Design review of the part built by this model. Coordinates are the model's own, in mm. Face numbers are marked on the shaded views. A direction names the side the tool comes from. Coordinates: 2 decimals unless noted, no trailing zeros. Write each loop counter-clockwise with the first axis right and the second up, starting at its lowest first coordinate (ties: lowest second). Pieces come first, ordered by that corner, then holes. Notation, with made-up numbers: (-23.5, 15.25) - (21.5, 15.25) arc R31 ccw to (21.5, 51.25) - close; hole circle Ø2 at (-33, -25). An arc over 180 degrees is marked (long way). Use a Markdown table: item, result.
from build123d import *

# Parameters (mm, degrees)
SKETCH1_W           = 30
SKETCH1_H           = 28
BOSS_EXTRUDE1_DEPTH = 20
SKETCH2_W           = 5
SKETCH2_H           = 28
BOSS_EXTRUDE2_DEPTH = 12
SKETCH3_W           = 3
SKETCH3_H           = 2
CUT_EXTRUDE1_DEPTH  = 53.038447325
SKETCH4_W           = 20
SKETCH4_H           = 20
CUT_EXTRUDE2_DEPTH  = 14
SKETCH5_W           = 7
SKETCH5_H           = 2
BOSS_EXTRUDE3_DEPTH = 28
FILLET1_R           = 2
BOSS_EXTRUDE5_DEPTH = 10
SKETCH8_W           = 26
SKETCH8_H           = 2
BOSS_EXTRUDE6_DEPTH = 8.8
BOSS_EXTRUDE7_DEPTH = 4


with BuildPart() as part:
    # Sketch1 → Boss-Extrude1 (new body)
    with BuildSketch(Plane(origin=(0, 0, 0), x_dir=(1, 0, 0), z_dir=(0, 1, 0))):
        with Locations((-15, 14)):
            Rectangle(SKETCH1_W, SKETCH1_H)
    extrude(amount=BOSS_EXTRUDE1_DEPTH)

    # Sketch2 → Boss-Extrude2 (add)
    with BuildSketch(Plane(origin=(0, 20, 0), x_dir=(1, 0, 0), z_dir=(0, 1, 0))):
        with Locations((-27.5, 14)):
            Rectangle(SKETCH2_W, SKETCH2_H)
        with Locations((-2.5, 14)):
            Rectangle(SKETCH2_W, SKETCH2_H)
    extrude(amount=BOSS_EXTRUDE2_DEPTH)

    # Sketch3 → Cut-Extrude1 (cut, through all)
    with BuildSketch(Plane.XY):
        with Locations((-3.5, 21)):
            Rectangle(SKETCH3_W, SKETCH3_H)
        with Locations((-26.5, 21)):
            Rectangle(SKETCH3_W, SKETCH3_H)
    extrude(amount=-CUT_EXTRUDE1_DEPTH, mode=Mode.SUBTRACT)

    # Sketch4 → Cut-Extrude2 (cut)
    with BuildSketch(Plane.XY):
        with Locations((-15, 10)):
            Rectangle(SKETCH4_W, SKETCH4_H)
    extrude(amount=-CUT_EXTRUDE2_DEPTH, mode=Mode.SUBTRACT)

    # Sketch5 → Boss-Extrude3 (add)
    with BuildSketch(Plane(origin=(0, 0, -28), x_dir=(-1, 0, 0), z_dir=(0, 0, -1))):
        with Locations((33.5, 1)):
            Rectangle(SKETCH5_W, SKETCH5_H)
        with Locations((-3.5, 1)):
            Rectangle(SKETCH5_W, SKETCH5_H)
    extrude(amount=-BOSS_EXTRUDE3_DEPTH)

    # Fillet1
    fillet1_edges = [part.edges().sort_by_distance(p)[0] for p in [
        (-30, 2, -14),
        (0, 2, -14),
    ]]
    fillet(fillet1_edges, radius=FILLET1_R)

    # Sketch7 → Boss-Extrude5 (add)
    with BuildSketch(Plane(origin=(0, 32, 0), x_dir=(1, 0, 0), z_dir=(0, 1, 0))):
        with BuildLine():
            Line((-25, 15), (-25, 28))
            Line((-25, 28), (-5, 28))
            Line((-5, 28), (-5, 15))
            ThreePointArc((-5, 15), (-15, 25), (-25, 15))
        make_face()
    extrude(amount=-BOSS_EXTRUDE5_DEPTH)

    # Sketch8 → Boss-Extrude6 (add)
    with BuildSketch(Plane(origin=(0, 0, -28), x_dir=(-1, 0, 0), z_dir=(0, 0, -1))):
        with Locations((15, 21)):
            Rectangle(SKETCH8_W, SKETCH8_H)
    extrude(amount=-BOSS_EXTRUDE6_DEPTH)

    # Sketch10 → Boss-Extrude7 (add)
    with BuildSketch(Plane(origin=(0, 0, -28), x_dir=(-1, 0, 0), z_dir=(0, 0, -1))):
        with BuildLine():
            Line((30, 4), (30, 32))
            Line((30, 32), (0, 32))
            Line((0, 32), (0, 4))
            ThreePointArc((0, 4), (-0.585786438, 2.585786438), (-2, 2))
            Line((-2, 2), (-7, 2))
            Line((-7, 2), (-7, 0))
            Line((-7, 0), (37, 0))
            Line((37, 0), (37, 2))
            Line((37, 2), (32, 2))
            ThreePointArc((32, 2), (30.585786438, 2.585786438), (30, 4))
        make_face()
    extrude(amount=BOSS_EXTRUDE7_DEPTH)


solid = part.part
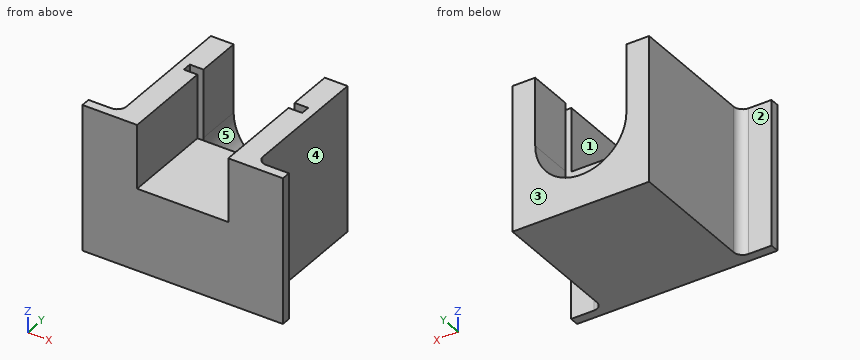
(1) Machinability: for the marked faces 1, 2, 3, 4 and 5, which of the approach directions +Z, -Z, +X, -X, +Y, -Y give a long, thin tool a straight path to every point of the face, cutting with its end or side? Answer none if there is none.
Determined:
| item | result |
|---|---|
| face 1 | +Z, +Y, -Y |
| face 2 | +Z, -Z, -X, +Y |
| face 3 | +Z, -Z, +X, -X, +Y |
| face 4 | +Z, -Z, +X, +Y |
| face 5 | +Z, +Y |
(2) For pin 1 (15.5 mm diameter, centred on y = 13.5, z = -6.5, fed in from -X); pin 2 (1.6 mm diameter, centred on x = -18, y = 21, fed in from +Z); pin 3 (1 mm diameter, centred on y = 20.5, z = -12, fed in from +X), all flat-tipped, find the tip position at first contact; note any pin that passes through.
Determined:
| item | result |
|---|---|
| pin 1 | x = -30 |
| pin 2 | z = -19.2 |
| pin 3 | x = 0 |
(3) Take a section at C-C on z = -21. Write out the cut boundary in (x, y), and give its area (3 significant figures).
Determined:
| item | result |
|---|---|
| outline | (-37, 0) - (7, 0) - (7, 2) - (2, 2) arc R2 cw to (0, 4) - (0, 32) - (-7, 32) - (-7, 22) - (-23, 22) - (-23, 32) - (-30, 32) - (-30, 4) arc R2 cw to (-32, 2) - (-37, 2) - close |
| area | 830 mm2 |
(4) Take a section at A-A on z = -11. Write out the cut boundary in (x, y), and give its area (3 significant figures).
Determined:
| item | result |
|---|---|
| outline | (-37, 0) - (-25, 0) - (-25, 20) - (-28, 20) - (-28, 22) - (-25, 22) - (-25, 32) - (-30, 32) - (-30, 4) arc R2 cw to (-32, 2) - (-37, 2) - close; (-5, 0) - (7, 0) - (7, 2) - (2, 2) arc R2 cw to (0, 4) - (0, 32) - (-5, 32) - (-5, 22) - (-2, 22) - (-2, 20) - (-5, 20) - close |
| area | 338 mm2 |
(5) For L1, parallel to X at y = 12.5, z = -2; L2, parallel to X at y = 21, z = -15.5; L3, parallel to Z at x = -21.5, y = 14.5, list the stretches that pass through material, from the lowest coordinate up. Write a range as from..to.
Determined:
| item | result |
|---|---|
| L1 | -30..-25, -5..0 |
| L2 | -30..-28, -2..0 |
| L3 | -32..-14 |
(6) Take a section at D-D on x = -15. Write out the cut boundary in (y, z), and give its area (3 significant figures).
Determined:
| item | result |
|---|---|
| outline | (0, -32) - (32, -32) - (32, -25) - (22, -25) - (22, -19.2) - (20, -19.2) - (20, -14) - (0, -14) - close |
| area | 456 mm2 |
(7) Take a section at B-B on y = 13.5. Write out the cut boundary in (x, z).
Determined:
| item | result |
|---|---|
| outline | (-30, -32) - (0, -32) - (0, 0) - (-5, 0) - (-5, -14) - (-25, -14) - (-25, 0) - (-30, 0) - close |
